Here's the drawing with two shaded views (mm, measured from the low corner). I have some questions. A direction names the side the tool comes from. Round coordinates to 2 decimals unless told otherwise and drop trailing zeros. Order: outer loops, then holes, each group sorted by start corner. A loop starts at its lowest first (then second) coordinate and runs counter-clockwise, first axis right, second up. Notation, with made-up numbers: M 67,-31 L 96,-31 A20 cw 96,-2 Z; hole C 46,4 d2. An arc over 180 degrees is marked long. One line per question, with ' | ' between items.
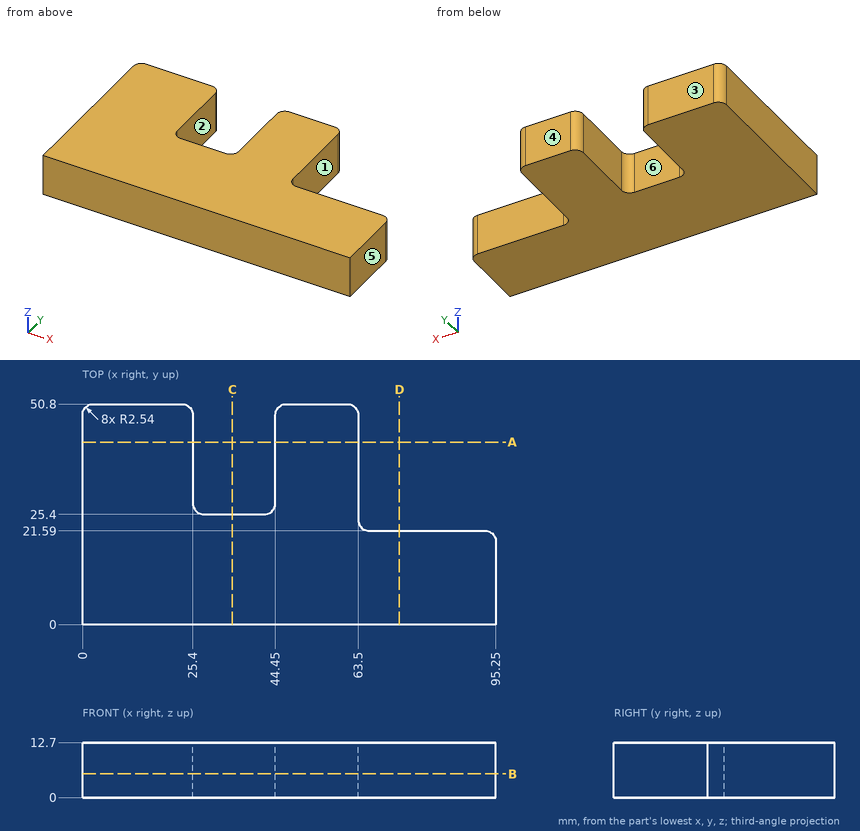
(1) Will these pins go through, and if not, where does the flat tip stop? pin 1 Ø4 at (y, z) = (31.5, 8) entering from +X; pin 2 Ø4 at (x, z) = (36.5, 8) entering from +Y; pin 3 Ø4 at (x, z) = (83.5, 6) entering from +Y.
Final values:
pin 1: x = 63.5 | pin 2: y = 25.4 | pin 3: y = 21.59
(2) If we section it at B-B on z = 5.5: Please give me the cut outline in (x, y), plus the area to 3 significant figures.
Final values:
outline: M 0,0 L 95.25,0 L 95.25,19.05 A2.54 ccw 92.71,21.59 L 66.04,21.59 A2.54 cw 63.5,24.13 L 63.5,48.26 A2.54 ccw 60.96,50.8 L 46.99,50.8 A2.54 ccw 44.45,48.26 L 44.45,27.94 A2.54 cw 41.91,25.4 L 27.94,25.4 A2.54 cw 25.4,27.94 L 25.4,48.26 A2.54 ccw 22.86,50.8 L 2.54,50.8 A2.54 ccw 0,48.26 Z | area: 3,420 mm^2
(3) Please list where these lines run through material, in increasing order: probe 1 along X at (y, z) = (48.5, 10.5); probe 2 along X at (y, z) = (41.5, 2.5); probe 3 along Y at (x, z) = (31, 10). Write a range as [from, to].
Final values:
probe 1: [0.01, 25.39], [44.46, 63.49] | probe 2: [0, 25.4], [44.45, 63.5] | probe 3: [0, 25.4]
(4) If we section it at C-C on x = 34.5: Please give me the cut outline in (y, z), plus the area to 3 significant figures.
Final values:
outline: M 0,0 L 25.4,0 L 25.4,12.7 L 0,12.7 Z | area: 323 mm^2
(5) If we section it at D-D on x = 73: Please give me the cut outline in (y, z), plus the area to 3 significant figures.
Final values:
outline: M 0,0 L 21.59,0 L 21.59,12.7 L 0,12.7 Z | area: 274 mm^2
(6) Thinking about a two-plate mould opening in X: for the marked faces 4, 5 and 6, which applies, released by +X, released by -X, zero draft, split by the parting line, or undercut?
Final values:
face 4: zero draft | face 5: released by +X | face 6: undercut
(7) On a 3-axis mill with a long thin cutter (end or side, diameter ignored), from which of +Z, -Z, +X, -X, +Y, -Y can I reach the whole of each face in a straight line? I mean the marked faces 1, 2 and 3. Say none if no direction works.
Final values:
face 1: +Z, -Z, +X, +Y | face 2: +Z, -Z, +Y | face 3: +Z, -Z, +X, -X, +Y
(8) If we section it at A-A on y = 42: Please give me the cut outline in (x, z), plus the area to 3 significant figures.
Final values:
outline: M 0,0 L 25.4,0 L 25.4,12.7 L 0,12.7 Z; M 44.45,0 L 63.5,0 L 63.5,12.7 L 44.45,12.7 Z | area: 565 mm^2
